Autodesk Inventor part; units mm, degrees
ref_plane "Pracovní rovina1" through (0, 0, 20) normal (0, 0, 1) x (1, 0, 0)
ref_plane "YZ Plane" through (0, 0, 0) normal (1, 0, 0) x (0, 1, 0)
ref_plane "XZ Plane" through (0, 0, 0) normal (0, 1, 0) x (-1, 0, 0)
sketch "Náčrt1" plane through (0, 0, 0) normal (0, 0, 1) x (1, 0, 0)
  line L0 (2.5, -1.4434) -> (0, -2.8868)
  line L1 (0, -2.8868) -> (-2.5, -1.4434)
  line L2 (-2.5, -1.4434) -> (-2.5, 1.4434)
  line L3 (-2.5, 1.4434) -> (0, 2.8868)
  line L4 (0, 2.8868) -> (2.5, 1.4434)
  line L5 (2.5, 1.4434) -> (2.5, -1.4434)
  circle A0 centre (0, 0) radius 1.5
  point P0 (2.5, 0)
  dimension "d1" = 3
  dimension "d16" = 5
extrude "Vysunutí1" add sketch "Náčrt1" along normal blind 40
thread "Závit1"
sketch "Náčrt2" plane through (0, 0, 40) normal (0, 0, 1) x (1, 0, 0)
  circle A0 centre (0, 0) radius 2.5
  dimension "d18" = 5
extrude "Vysunutí2" cut sketch "Náčrt2" against normal through all draft 45 keep common part
sketch "Náčrt3" plane through (0, 0, 0) normal (0, 0, -1) x (-1, 0, 0)
  circle A0 centre (0, 0) radius 2.5
  dimension "d17" = 5
extrude "Vysunutí3" cut sketch "Náčrt3" against normal through all draft 45 keep common part
chamfer "Zkosení1" distance 0.2 angle 45 1 edges at (-1.5, 0, 40)
chamfer "Zkosení2" distance 0.2 angle 45 1 edges at (-1.5, 0, 0)
ref_plane "Pracovní rovina1" through (0, 0, 20) normal (0, 0, 1) x (1, 0, 0)
sketch "Náčrt4" plane through (0, 0, 20) normal (0, 0, 1) x (1, 0, 0)
  point P0 (0, 0)
sketch "Náčrt5" plane through (0, 0, 20) normal (0, 0, 1) x (1, 0, 0)
  circle A0 centre (0, 0) radius 1.5
  dimension "d19" = 3
extrude "Vysunutí4" add sketch "Náčrt5" along normal mid plane 18
properties part number "PillarBolt-M3x40" material "Ocel, vysokopevnostní, nízkolegovaná"
Part model, mm, in its own coordinate system. A direction names the side the tool comes from. Round coordinates to 2 decimals unless told otherwise and drop trailing zeros. Loops run counter-clockwise (first coordinate to the right, second up) from the corner with the lowest first, then second, coordinate; pieces in that order, holes last. Notation, with made-up numbers: (21.25, -35.75) -> (25.25, -35.75) arc R15 ccw to (25.25, -28.75) -> close; hole circle Ø8 at (55.5, -5). An arc over 180 degrees is marked (long way). Use one line per item in the form item = value. Start each with the question number.
Item 1: Drop flat-ended pins along their axis: pin 1 Ø3 at (y, z) = (2, 8) entering from -X; pin 2 Ø1.5 at (x, y) = (-0.5, 0.5) entering from -Z; pin 3 Ø1 at (x, z) = (-1.5, 28) entering from +Y. Give the stop position or say it passes through.
Item 2: Drill centre lines: line 1 along Z through (x, y) = (1.1, 0.95); line 2 along Y through (x, z) = (-0.55, 31.5); line 3 along Y through (x, z) = (-0.25, 32.5). Where is each one in solid material? Low to high.
Item 3: Band-saw the part on A-A (z = 33). List the corners of the cut face in (x, y).
Item 4: Two-plate mould, pull along Y, no slides. Class faces 1 (the cylindrical face through (-1.5, -0.07, 5.52)), 2 (the conical face through (2.29, 1.31, 0.14)), 3 (the conical face through (-2.268, -1.317, 39.877)): released by +Y, released by -Y, zero draft, split by the parting line, or undercut.
Item 5: Band-saw the part on B-B (z = 19). List the corners of the cut face in (x, y), plus the area to 3 significant figures.
Item 6: Tool access for faces 4 (the cylindrical face through (-1.5, -0.07, 34.32)), 5 (the flat face through (0, 0, 11)), 6 (the flat face through (-1.268, 2.155, 19.72)): list every direction of +Z, -Z, +X, -X, +Y, -Y with a clear straight run to the whole face (end or side of a thin tool).
Data:
q1.pin_1 = -2.5
q1.pin_2 = 11
q1.pin_3 = 2.31
q2.line_1 = 11 to 29
q2.line_2 = -2.57 to -1.4, 1.4 to 2.57
q2.line_3 = -2.74 to -1.48, 1.48 to 2.74
q3.outline = (-2.5, -1.44) -> (0, -2.89) -> (2.5, -1.44) -> (2.5, 1.44) -> (0, 2.89) -> (-2.5, 1.44) -> close; hole circle Ø3 at (0, 0)
q4.face_1 = undercut
q4.face_2 = released by +Y
q4.face_3 = released by -Y
q5.outline = (-2.5, -1.44) -> (0, -2.89) -> (2.5, -1.44) -> (2.5, 1.44) -> (0, 2.89) -> (-2.5, 1.44) -> close
q5.area = 21.7 mm^2
q6.face_4 = +Z
q6.face_5 = -Z
q6.face_6 = +Z, -Z, -X, +Y
